Geometry: see drawing. Coordinates: mm, zero at the bounding-box minimum. Round coordinates to 2 decimals unless told otherwise and drop trailing zeros. Order: outer loops, then holes, each group sorted by start corner. A loop starts at its lowest first (then second) coordinate and runs counter-clockwise, first axis right, second up.
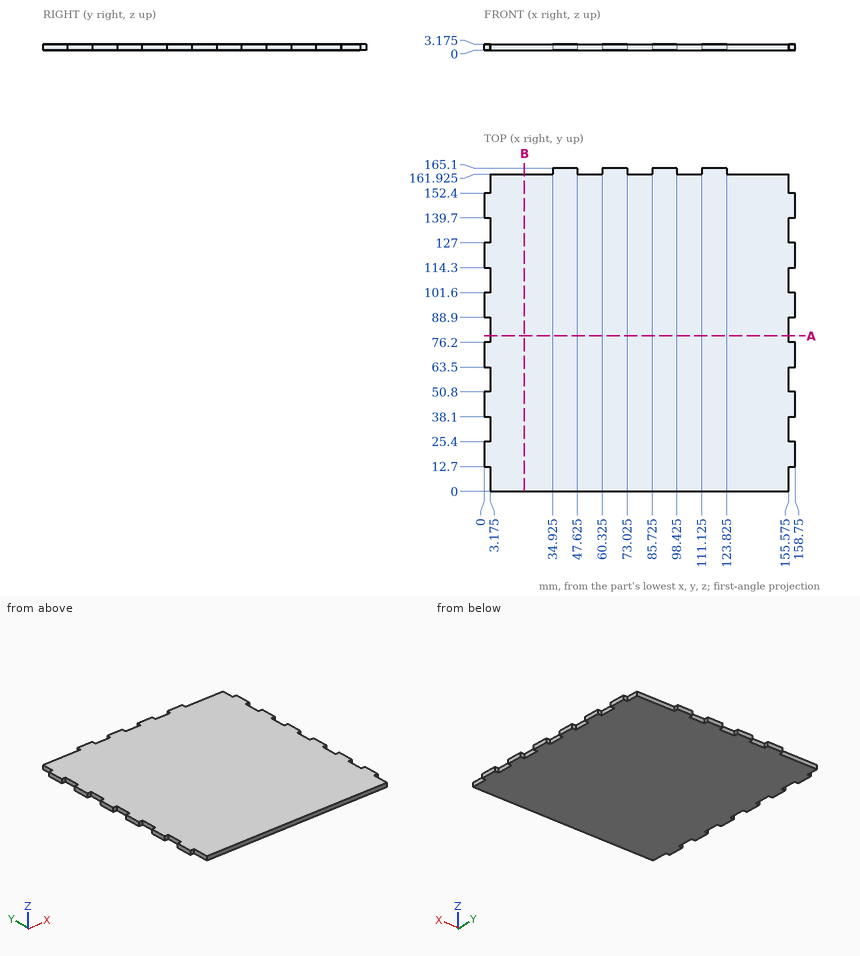
1. Section A-A on y = 79.5. Return loops of the section in (x, z) (3 decimals).
2. Line query: line 1 along X through (y, z) = (61, 0.25) (3 decimals); line 2 along Y through (x, z) = (104.5, 1.3) (3 decimals). Output: solid intervals per line, ascending.
3. First-contact query: pin 1 (1 mm diameter, centred on y = 57.5, z = 1, fed in from +X) (3 decimals); pin 2 (1 mm diameter, centred on x = 157, z = 1.5, fed in from +Y); pin 3 (1 mm diameter, centred on x = 157.5, z = 2.5, fed in from -Y). Flat tips, straight axial feed; report the tip coordinate or a pass-through.
4. Section B-B on x = 20.5. Return loops of the section in (y, z) (3 decimals), plus the area to 3 significant figures.
Result:
1. outline: (3.175, 0) - (155.575, 0) - (155.575, 3.175) - (3.175, 3.175) - close
2. line 1: x = 3.175 to 155.575
2. line 2: y = 0 to 161.925
3. pin 1: stops at x = 155.575
3. pin 2: stops at y = 152.4
3. pin 3: stops at y = 12.7
4. outline: (0, 0) - (161.925, 0) - (161.925, 3.175) - (0, 3.175) - close
4. area: 514 mm2
